from build123d import *

# Parameters (mm, degrees)
CUT_EXTRUDE1_DEPTH = 5.5
CHAMFER2_SIZE      = 2


with BuildPart() as part:
    # Sketch1 → Revolve1 (revolve)
    with BuildSketch(Plane.XY):
        Polygon((0, 0), (0, 18), (28, 18), (28, 23), (78, 23), (78, 29), (88, 29), (88, 21), (138, 21), (138, 0), align=None)
    revolve(axis=Axis((0, 0, 0), (1, 0, 0)))

    # Sketch2 → Cut-Extrude1 (cut)
    with BuildSketch(Plane.XY.offset(23)):
        with BuildLine():
            Line((41, 7), (65, 7))
            ThreePointArc((65, 7), (72, 0), (65, -7))
            Line((65, -7), (41, -7))
            ThreePointArc((41, -7), (34, 0), (41, 7))
        make_face()
    extrude(amount=-CUT_EXTRUDE1_DEPTH, mode=Mode.SUBTRACT)

    # Chamfer2
    chamfer2_edges = [part.edges().sort_by_distance(p)[0] for p in [
        (0, -18, 0),
        (138, -21, 0),
    ]]
    chamfer(chamfer2_edges, length=CHAMFER2_SIZE)


solid = part.part
Can you work these out from the model? Positions are in its coordinate system, mm. A direction names the side the tool comes from. Coordinates: 2 decimals unless noted, no trailing zeros. Order: outer loops, then holes, each group sorted by start corner. A loop starts at its lowest first (then second) coordinate and runs counter-clockwise, first axis right, second up. Notation, with made-up numbers: (40, -32) - (94, -32) arc R27 ccw to (94, 3) - close; hole circle Ø5 at (19.5, -1.75). An arc over 180 degrees is marked (long way). Answer as a JSON object with one key per item and string values. Group by question number.
Q1. Imagine slicing it at D-D (x = 90.5). Please give me the cut outline in (y, z), and give its area (3 significant figures).
Q2. I need wall thicknesses on line 1 (Y direction, x = 79.5, z = -1); line 2 (Z direction, x = 87, y = -0.5); line 3 (X direction, y = -17, z = -22). Which ranges of each line are inside material? Lowest first, please. Write a range as from..to.
Q3. Imagine slicing it at A-A (z = 0). Please give me the cut outline in (x, y).
Q4. On a 3-axis mill with a long thin cutter (end or side, diameter ignored), from which of +Z, -Z, +X, -X, +Y, -Y can I reach the whole of each face in a straight line? I mean faces 4 (the face through (53.35, -4.986, -22.453)), 5 (the face through (112.34, 20.03, 6.31)), 6 (the face through (53, -7, 20)). Say none if no direction works.
Q5. Imagine slicing it at C-C (x = 10). Please give me the cut outline in (y, z), and give its area (3 significant figures).
Q6. Will these pins go through, and if not, where does the flat tip stop? P1, Ø6, axis at x = 53.5, z = -17.5, coming from the +Y side; P2, Ø1, axis at x = 85.5, y = -3.5, coming from the +Z side; P3, Ø6, axis at x = 15, z = -14.5, coming from the +Y side; P4, Ø8, axis at y = 14.5, z = -12, coming from the -X side.
Q7. We'd pull the mould along Y, two halves only. Please class faces 1 (the face through (72, 0, 20)), 2 (the face through (15.182, -2.343, 17.847)), 3 (the face through (78, 9, 22)): +Y half, -Y half, draft (parallel to the pull), parting line (faces both ways), or undercut.
Q8. Imagine slicing it at B-B (y = 0). Please give me the cut outline in (x, z), and give its area (3 significant figures).
Determined:
{
 "1": {"outline": "circle Ø42 at (0, 0)", "area": "1,390 mm2"},
 "2": {"line 1": "y = -28.98..28.98", "line 2": "z = -29..29", "line 3": "x = 78..88"},
 "3": {"outline": "(0, -16) - (2, -18) - (28, -18) - (28, -23) - (78, -23) - (78, -29) - (88, -29) - (88, -21) - (136, -21) - (138, -19) - (138, 19) - (136, 21) - (88, 21) - (88, 29) - (78, 29) - (78, 23) - (28, 23) - (28, 18) - (2, 18) - (0, 16) - close"},
 "4": {"face 4": "-X", "face 5": "+X", "face 6": "+Z"},
 "5": {"outline": "circle Ø36 at (0, 0)", "area": "1,020 mm2"},
 "6": {"P1": "stops at y = 17.85", "P2": "stops at z = 28.84", "P3": "stops at y = 13.85", "P4": "stops at x = 0"},
 "7": {"face 1": "undercut", "face 2": "parting line", "face 3": "draft"},
 "8": {"outline": "(0, -16) - (2, -18) - (28, -18) - (28, -23) - (78, -23) - (78, -29) - (88, -29) - (88, -21) - (136, -21) - (138, -19) - (138, 19) - (136, 21) - (88, 21) - (88, 29) - (78, 29) - (78, 23) - (72, 23) - (72, 17.5) - (34, 17.5) - (34, 23) - (28, 23) - (28, 18) - (2, 18) - (0, 16) - close", "area": "5,770 mm2"}
}
